```python
from build123d import *

# Parameters (mm, degrees)
BOSS_EXTRUDE1_DEPTH      = 11
BOSS_EXTRUDE1_DEPTH_BACK = 11
CUT_EXTRUDE1_DEPTH       = 23.154288524
CUT_EXTRUDE1_DEPTH_BACK  = 23.154288524
SKETCH2_R                = 1.75
CUT_EXTRUDE2_REACH       = 25.718
SKETCH3_R                = 1.5
FILLET1_R                = 1
CHAMFER1_SIZE            = 0.75


with BuildPart() as part:
    # Sketch1 → Boss-Extrude1 (new, two sides: drawn at the far end of the back side and taken through both)
    with BuildSketch(Plane(origin=(0, 0, 0), x_dir=(1, 0, 0), z_dir=(0, 1, 0)).offset(-BOSS_EXTRUDE1_DEPTH_BACK)):
        with BuildLine():
            Line((-15.25, 0), (-15.25, -5))
            ThreePointArc((-15.25, -5), (-14.810660172, -6.060660172), (-13.75, -6.5))
            Line((-13.75, -6.5), (13.75, -6.5))
            ThreePointArc((13.75, -6.5), (14.810660172, -6.060660172), (15.25, -5))
            Line((15.25, -5), (15.25, 0))
            Line((15.25, 0), (15.25, 3.5))
            Line((15.25, 3.5), (17.25, 3.5))
            Line((17.25, 3.5), (17.25, 0))
            Line((17.25, 0), (17.25, -5))
            ThreePointArc((17.25, -5), (16.224873734, -7.474873734), (13.75, -8.5))
            Line((13.75, -8.5), (-13.75, -8.5))
            ThreePointArc((-13.75, -8.5), (-16.224873734, -7.474873734), (-17.25, -5))
            Line((-17.25, -5), (-17.25, 0))
            Line((-17.25, 0), (-17.25, 3.5))
            Line((-17.25, 3.5), (-15.25, 3.5))
            Line((-15.25, 3.5), (-15.25, 0))
        make_face()
    extrude(amount=BOSS_EXTRUDE1_DEPTH + BOSS_EXTRUDE1_DEPTH_BACK)

    # Sketch2 → Cut-Extrude1 (cut, two sides: drawn at the far end of the back side and taken through both)
    with BuildSketch(Plane(origin=(0, 0, 0), x_dir=(0, 0, -1), z_dir=(1, 0, 0)).offset(-CUT_EXTRUDE1_DEPTH_BACK)):
        with Locations((0, 7.5)):
            Circle(SKETCH2_R)
        with Locations((0, -7.5)):
            Circle(SKETCH2_R)
    extrude(amount=CUT_EXTRUDE1_DEPTH + CUT_EXTRUDE1_DEPTH_BACK, mode=Mode.SUBTRACT)

    # Sketch3 → Cut-Extrude2 (cut, up to next)
    with BuildSketch(Plane.XY.offset(8.5), mode=Mode.PRIVATE) as cut_extrude2_sk1:
        Circle(SKETCH3_R)
    cut_extrude2_tool1 = extrude(cut_extrude2_sk1.sketch, amount=-CUT_EXTRUDE2_REACH, mode=Mode.PRIVATE) & part.part
    add(cut_extrude2_tool1.solids().sort_by_distance((0, 0, 8.5))[0], mode=Mode.SUBTRACT)

    # Fillet1
    fillet1_edges = [part.edges().sort_by_distance(p)[0] for p in [
        (-16.25, -11, -3.5),
        (-17.25, -11, 0.75),
        (-16.224873734, -11, 7.474873734),
        (0, -11, 8.5),
        (15.25, 0, -3.5),
        (17.25, 0, -3.5),
        (-17.25, 0, -3.5),
        (-15.25, 0, -3.5),
        (16.224873734, -11, 7.474873734),
        (17.25, -11, 0.75),
        (16.25, -11, -3.5),
        (-14.810660172, -11, 6.060660172),
        (15.25, -11, 0.75),
        (-14.810660172, 11, 6.060660172),
        (-15.25, 11, 0.75),
        (-16.25, 11, -3.5),
        (-17.25, 11, 0.75),
        (14.810660172, -11, 6.060660172),
        (-16.224873734, 11, 7.474873734),
        (0, 11, 8.5),
        (16.224873734, 11, 7.474873734),
        (17.25, 11, 0.75),
        (16.25, 11, -3.5),
        (15.25, 11, 0.75),
        (14.810660172, 11, 6.060660172),
        (0, 11, 6.5),
        (0, -11, 6.5),
        (-15.25, -11, 0.75),
    ]]
    fillet(fillet1_edges, radius=FILLET1_R - 0.0001)  # a hair under: the kernel refuses the full size

    # Chamfer1
    chamfer1_edges = [part.edges().sort_by_distance(p)[0] for p in [
        (-17.25, 7.5, 1.75),
        (17.25, 7.5, 1.75),
        (-17.25, -7.5, 1.75),
        (17.25, -7.5, 1.75),
    ]]
    chamfer(chamfer1_edges, length=CHAMFER1_SIZE)


solid = part.part
```
Source: CAD feature listing. Evaluate the final solid. Frame: model axes, mm. A direction names the side the tool comes from. Round coordinates to 2 decimals unless told otherwise and drop trailing zeros. Answer as a JSON object with one key per item and string values. Group by question number.
(1) First-contact query: pin 1 (12 mm diameter, centred on x = 5, y = 4.5, fed in from -Z); pin 2 (2.5 mm diameter, centred on x = 0, y = 0, fed in from -Z). Flat tips, straight axial feed; report the tip coordinate or a pass-through.
(2) Reachability of faces 1 (the cylindrical face through (16.949, 10.715, 1.302)), 2 (the cylindrical face through (-14.82, -0.14, 6.05)), 3 (the cylindrical face through (0.193, -10.699, 6.785)) from +Z, -Z, +X, -X, +Y, -Y: full face, straight path, thin tool, end or side. Return the list, or none.
(3) Mould query, pull axis X, two halves, no side actions, for faces 4 (the flat face through (17.25, 0, 2)), 5 (the cylindrical face through (15.535, 0.14, -3.199)), 6 (the cylindrical face through (-15.88, -9.21, 0.38)). Classes: +X half, -X half, draft (parallel to the pull), parting line (faces both ways), or undercut.
(4) Section query A-A on y = -7.5. State how many separate pieces and enclosed holes the cut face has, then the cut area to 3 significant figures.
(5) Ray query, line 1 (X direction, y = -5.75, z = 4.5); line 2 (Y direction, x = -15.65, z = 0); line 3 (Z direction, x = -3, y = -9.5). Return the intervals inside material, ascending. Write a range as [from, to].
Computed values:
{
 "1": {"pin 1": "z = 6.5", "pin 2": "through"},
 "2": {"face 1": "+Z, -Z, +X, +Y", "face 2": "-Z, +Y, -Y", "face 3": "-Z, -Y"},
 "3": {"face 4": "+X half", "face 5": "undercut", "face 6": "draft"},
 "4": {"separate pieces": "3", "enclosed holes": "0", "area": "88.7 mm^2"},
 "5": {"line 1": "[-17.25, -15.25], [15.25, 17.25]", "line 2": "[-10.8, -9.25], [-5.75, 5.75], [9.25, 10.8]", "line 3": "[6.5, 8.5]"}
}
